from build123d import *

# Parameters (mm, degrees)
F0_W = 8.33
F0_H = 12.5


with BuildPart() as f1:
    # F0 (on Front) → F1 (revolve)
    with BuildSketch(Plane.XZ):
        with BuildLine():
            Line((-8.4, 0), (0, 0))
            Line((0, 0), (0, 6.01))
            ThreePointArc((0, 6.01), (-0.146447, 6.363553), (-0.5, 6.51))
            Line((-0.5, 6.51), (-8.4, 6.51))
            Line((-8.4, 6.51), (-8.4, 0))
        make_face()
        Polygon((-10.322576, 0), (-8.4, 0), (-8.4, 6.51), (-10.322576, 5.4), align=None)
        Polygon((-19.67, 0), (-10.322576, 0), (-10.322576, 5.4), (-14.319766, 5.4), (-19.67, 12.5), align=None)
        with Locations((-23.835, 6.25)):
            Rectangle(F0_W, F0_H)
    revolve(axis=Axis((-14, 0, 0), (1, 0, 0)))


solid = f1.part
CAD build for the part. Positions are in the model's coordinates, mm. A direction names the side the tool comes from. Round coordinates to 2 decimals unless told otherwise and drop trailing zeros. Write each loop counter-clockwise with the first axis right and the second up, starting at its lowest first coordinate (ties: lowest second). Pieces come first, ordered by that corner, then holes.
(1) Slice it at D-D, the plane x = -17.75. Write the cut outline in (y, z).
(2) Slice it at C-C, the plane x = -1.25. Write the cut outline in (y, z).
(3) Slice it at A-A, the plane z = 0. Write the cut outline in (x, y).
(4) Drop flat-ended pins along their axis: P1, Ø1, axis at x = -18.5, y = 8, coming from the +Z side; P2, Ø1.5, axis at x = -20, z = -5, coming from the +Y side; P3, Ø4, axis at x = -16.5, z = 7.5, coming from the +Y side. Give the stop position or say it passes through.
(5) Probe line 1 along X through (y, z) = (-2, 5.75); line 2 along Y through (x, z) = (-14.25, -0.25); line 3 along Y through (x, z) = (-18, 1). List the from-to ranges inside material, lowest first.
(6) 3-axis set-ups, long thin cutter, end or side, ignore diameter. For faces 1 (the face through (-4.505, 2.493, 6.014)), 2 (the face through (-12.35, 5.27, -1.17)), 3 (the face through (0, 0, 0)): which of +Z, -Z, +X, -X, +Y, -Y reach the whole face in a straight line?
From the geometry:
1. outline: circle Ø19.9 at (0, 0)
2. outline: circle Ø13.02 at (0, 0)
3. outline: (-28, -12.5) - (-19.67, -12.5) - (-14.32, -5.4) - (-10.32, -5.4) - (-8.4, -6.51) - (-0.5, -6.51) arc R0.5 ccw to (0, -6.01) - (0, 6.01) arc R0.5 ccw to (-0.5, 6.51) - (-8.4, 6.51) - (-10.32, 5.4) - (-14.32, 5.4) - (-19.67, 12.5) - (-28, 12.5) - close
4. P1: stops at z = 8.53
4. P2: stops at y = 11.76
4. P3: stops at y = 8.38
5. line 1: x = -28 to -14.84, -9.13 to -0.01
5. line 2: y = -5.39 to 5.39
5. line 3: y = -10.24 to 10.24
6. face 1: +X
6. face 2: none
6. face 3: +Z, -Z, +X, +Y, -Y
